Read the model definition and answer for the solid it produces. Units are mm, in the model's axes. A direction names the side the tool comes from. Give positions to 0.01 mm unless a question says otherwise; leave off trailing zeros. Order: outer loops, then holes, each group sorted by start corner. A loop starts at its lowest first (then second) coordinate and runs counter-clockwise, first axis right, second up.
```python
from build123d import *

# Parameters (mm, degrees)
PAD004_DEPTH    = 10
PAD005_DEPTH    = 20
PAD006_DEPTH    = 20
FILLET_R        = 5
SKETCH017_R     = 5
POCKET008_DEPTH = 13.75
POCKET009_DEPTH = 13.75
SKETCH019_R     = 3.175
POCKET010_DEPTH = 264.6116677124
POCKET011_DEPTH = 264.6116677124
POCKET012_DEPTH = 58
CHAMFER003_SIZE = 3
FILLET001_R     = 2
CHAMFER004_SIZE = 1


with BuildPart() as part:
    # Sketch014 → Pad004 (new body, symmetric)
    with BuildSketch(Plane.XY):
        with BuildLine():
            ThreePointArc((19.3, 0), (13.6471608769, 13.6471608769), (0, 19.3))
            Line((0, 19.3), (0, 25.3))
            ThreePointArc((25.3, 0), (17.889801564, 17.889801564), (0, 25.3))
            Line((19.3, 0), (25.3, 0))
        make_face()
    pad004 = extrude(amount=PAD004_DEPTH, both=True)

    # Mirrored007: Pad004 across Sketch014 H_Axis
    add(pad004.mirror(Plane.ZX))

    # Sketch015 (on Face4 of Mirrored007) → Pad005 (join)
    with BuildSketch(Plane.XY.offset(10)):
        with BuildLine():
            Line((0, 25.3), (0, 37.3))
            Line((0, 37.3), (6, 37.3))
            Line((6, 37.3), (6, 24.5782424107))
            ThreePointArc((6, 24.5782424107), (3.021627625, 25.1189125261), (0, 25.3))
        make_face()
    pad005 = extrude(amount=-PAD005_DEPTH)

    # Mirrored008: Pad005 across Sketch015 H_Axis
    add(pad005.mirror(Plane(origin=(0, 0, 10), x_dir=(0, 0, 1), z_dir=(0, 1, 0))))

    # Sketch016 (on Face8 of Mirrored008) → Pad006 (join)
    with BuildSketch(Plane.XY.offset(10)):
        with BuildLine():
            Line((50.25, 0), (64, 0))
            Line((64, 0), (64, 9.9))
            ThreePointArc((64, 9.9), (62.0528467529, 15.9796404149), (56.935983439, 19.7968570932))
            Line((6, 37.3), (56.935983439, 19.7968570932))
            Line((6, 37.3), (6, 24.5782424107))
            ThreePointArc((19.7996843409, 15.75), (13.6341627553, 21.3119592239), (6, 24.5782424107))
            Line((50.25, 15.75), (19.7996843409, 15.75))
            Line((50.25, 0), (50.25, 15.75))
        make_face()
    pad006 = extrude(amount=-PAD006_DEPTH)

    # Mirrored009: Pad006 across Sketch016 H_Axis
    add(pad006.mirror(Plane(origin=(0, 0, 10), x_dir=(0, 0, 1), z_dir=(0, 1, 0))))

    # Fillet
    fillet_edges = [part.edges().sort_by_distance(p)[0] for p in [
        (50.25, 15.75, 0),
        (50.25, -15.75, 0),
    ]]
    fillet(fillet_edges, radius=FILLET_R)

    # Sketch017 (on Face13 of Fillet) → Pocket008 (cut)
    with BuildSketch(Plane.YZ.offset(64)):
        Circle(SKETCH017_R)
    extrude(amount=-POCKET008_DEPTH, mode=Mode.SUBTRACT)

    # Sketch018 (on Face13 of Pocket008) → Pocket009 (cut)
    with BuildSketch(Plane.YZ.offset(64)):
        Polygon((-1.25, 4.8412291828), (-0.95, 5.1412291828), (0.95, 5.1412291828), (1.25, 4.8412291828), align=None)
    extrude(amount=-POCKET009_DEPTH, mode=Mode.SUBTRACT)

    # Sketch019 (on Face9 of Pocket009) → Pocket010 (cut, through all)
    with BuildSketch(Plane(origin=(0, 0, 0), x_dir=(0, -1, 0), z_dir=(-1, 0, 0))):
        with Locations((-31.3, 0)):
            Circle(SKETCH019_R)
    pocket010 = extrude(amount=-POCKET010_DEPTH, mode=Mode.SUBTRACT)

    # Mirrored010: Pocket010 across Sketch019 V_Axis
    add(pocket010.mirror(Plane(origin=(0, 0, 0), x_dir=(-1, 0, 0), z_dir=(0, -1, 0))), mode=Mode.SUBTRACT)

    # Sketch020 (on Face17 of Mirrored010) → Pocket011 (cut, through all)
    with BuildSketch(Plane(origin=(0, 0, 0), x_dir=(0, -1, 0), z_dir=(-1, 0, 0))):
        Polygon((-32.3, 3.0134075396), (-32.05, 3.2634075396), (-30.55, 3.2634075396), (-30.3, 3.0134075396), align=None)
    pocket011 = extrude(amount=-POCKET011_DEPTH, mode=Mode.SUBTRACT)

    # Mirrored011: Pocket011 across Sketch020 V_Axis
    add(pocket011.mirror(Plane(origin=(0, 0, 0), x_dir=(-1, 0, 0), z_dir=(0, -1, 0))), mode=Mode.SUBTRACT)

    # Sketch021 (on Face13 of Mirrored011) → Pocket012 (cut)
    with BuildSketch(Plane.YZ.offset(64)):
        with BuildLine():
            ThreePointArc((-31.3, -6), (-27.0573593129, -4.2426406871), (-25.3, 0))
            Line((-25.3, 10), (-25.3, 0))
            Line((-37.3, 10), (-25.3, 10))
            Line((-37.3, -6), (-37.3, 10))
            Line((-31.3, -6), (-37.3, -6))
        make_face()
    pocket012 = extrude(amount=-POCKET012_DEPTH, mode=Mode.SUBTRACT)

    # Mirrored012: Pocket012 across Sketch021 V_Axis
    add(pocket012.mirror(Plane(origin=(64, 0, 0), x_dir=(1, 0, 0), z_dir=(0, 1, 0))), mode=Mode.SUBTRACT)

    # Chamfer003
    chamfer003_edges = [part.edges().sort_by_distance(p)[0] for p in [
        (3, -37.3, 10),
        (3, 37.3, 10),
    ]]
    chamfer(chamfer003_edges, length=CHAMFER003_SIZE)

    # Fillet001
    fillet001_edges = [part.edges().sort_by_distance(p)[0] for p in [
        (19.799684, -15.75, 0),
        (19.799684, 15.75, 0),
    ]]
    fillet(fillet001_edges, radius=FILLET001_R)

    # Chamfer004
    chamfer004_edges = [part.edges().sort_by_distance(p)[0] for p in [
        (6, -37.3, 0.5),
        (6, -35.8, 8.5),
        (6, -29.8, 10),
        (23.46063, -25.3, 10),
        (48.928622, -22.548429, 10),
        (62.052847, -15.97964, 10),
        (64, 0, 10),
        (62.052847, 15.97964, 10),
        (48.928622, 22.548429, 10),
        (23.46063, 25.3, 10),
        (6, 29.8, 10),
        (6, 35.8, 8.5),
        (6, 37.3, 0.5),
        (21.850311, -14.74633, 10),
        (24.424003, -6.599853, 10),
        (24.424003, 6.599853, 10),
        (21.850311, 14.74633, 10),
        (34.417238, 15.75, 10),
        (48.785534, 14.285534, 10),
        (50.25, 0, 10),
        (48.785534, -14.285534, 10),
        (34.417238, -15.75, 10),
    ]]
    chamfer(chamfer004_edges, length=CHAMFER004_SIZE)


solid = part.part
```
1) The part is cut by section B-B on x = 28. Determine the outline of the cut face in (y, z), and give its area (3 significant figures).
Final values:
outline: (-29.74, -10) - (-15.75, -10) - (-15.75, 9) - (-16.75, 10) - (-24.3, 10) - (-25.3, 9) - (-25.3, 0) arc R6 cw to (-29.74, -5.79) - close; (15.75, -10) - (29.74, -10) - (29.74, -5.79) arc R6 cw to (25.3, 0) - (25.3, 9) - (24.3, 10) - (16.75, 10) - (15.75, 9) - close
area: 431 mm2
2) A tool of negligible diameter and unlimited length cuts with its end or side. For faces 1 (the face through (35, -15.75, 0)), 2 (the face through (48.946, 14.528, 9.285)), 3 (the face through (19.825, 27.104, -4.289)), 4 (the face through (12, -34, -6)), from which of +Z, -Z, +X, -X, +Y, -Y can it reach the whole face along a straight path? Write none if from no direction.
Final values:
face 1: +Z, -Z
face 2: +Z
face 3: +Z, +X, +Y
face 4: +Z, +X, -Y
3) Given pin 1 (1 mm diameter, centred on x = 50.5, y = 21, fed in from +Z); pin 2 (8 mm diameter, centred on y = 0, z = 0, fed in from +X); pin 3 (4 mm diameter, centred on x = 33, z = 0, fed in from +Y); pin 4 (3 mm diameter, centred on x = 13.5, y = -33.5, fed in from +Z), each flat-ended and moving along its own axis, determine where each tip first touches the part or whether it passes through.
Final values:
pin 1: stops at z = 10
pin 2: stops at x = 25.3
pin 3: stops at y = 25.64
pin 4: stops at z = -6
4) The part is cut by section A-A on x = 42. Determine the outline of the cut face in (y, z), and give its area (3 significant figures).
Final values:
outline: (-24.93, -10) - (-15.75, -10) - (-15.75, 9) - (-16.75, 10) - (-23.87, 10) - (-24.93, 9) - close; (15.75, -10) - (24.93, -10) - (24.93, 9) - (23.87, 10) - (16.75, 10) - (15.75, 9) - close
area: 365 mm2
5) For a pull along Y with two mould halves and no side action, classify faces 5 (the face through (57, 0, -5)), 6 (the face through (21.836, 14.721, -0.633)), 7 (the face through (6, -29.7, 3.3)), 8 (the face through (5.51, -35.46, 8.12)) as released by +Y, released by -Y, zero draft, split by the parting line, or undercut.
Final values:
face 5: undercut
face 6: undercut
face 7: zero draft
face 8: released by -Y
6) Consider L1, parallel to Y at x = 32.5, z = 5.5; L2, parallel to Y at x = 4.4, z = 0 (3 decimals); L3, parallel to Y at x = 22.5, z = 7.5. Determine where each line is inside the solid, lowest interval first.
Final values:
L1: y = -25.3 to -15.75, 15.75 to 25.3
L2: y = -37.3 to -34.475, -28.125 to -18.792, 18.792 to 28.125, 34.475 to 37.3
L3: y = -25.3 to -15.43, -11.57 to 11.57, 15.43 to 25.3
